Read the model definition and answer for the solid it produces. Units are mm, in the model's axes. Coordinates: 2 decimals unless noted, no trailing zeros. Write each loop counter-clockwise with the first axis right and the second up, starting at its lowest first coordinate (ties: lowest second). Pieces come first, ordered by that corner, then holes.
(1) Section D-D on z = 9 is taken. Write down the section's boundary in (x, y).
(2) Section C-C on y = -1.2 is taken. Write down the section's boundary in (x, z).
(3) Find the intervals of material crossed by probe 1 along X at (y, z) = (-0.7, 5); probe 2 along X at (y, z) = (1.25, 5.75); probe 3 along Z at (x, y) = (-10, -0.1), in increasing order.
(4) The mould has two halves that part along Z. Classify faces 1 (the cylindrical face through (8.753, -0.021, 3.373)), 2 (the flat face through (0, 0, 10)), 3 (the flat face through (0, 0, 0)), 4 (the cylindrical face through (0.09, -0.02, 2.95)): +Z half, -Z half, draft (parallel to the pull), parting line (faces both ways), or undercut.
(5) Given pin 1 (1.5 mm diameter, centred on y = 0, z = 6.5, fed in from -X); pin 2 (5.5 mm diameter, centred on x = 0, z = 5, fed in from +Y); pin 3 (3.5 mm diameter, centred on x = 10, z = 5, fed in from +Y), each flat-ended and moving along its own axis, determine where each tip first touches the part or whether it passes through.
(6) Section A-A on z = 5 is taken. Write down the section's boundary in (x, y).
(7) Section B-B on x = 0 is taken. Write down the section's boundary in (y, z).
from build123d import *

# Parameters (mm, degrees)
SKETCH1_R           = 2.05
BOSS_EXTRUDE1_DEPTH = 1.5


with BuildPart() as part:
    # Sketch1 → Boss-Extrude1 (new, symmetric)
    with BuildSketch(Plane(origin=(0, 0, 0), x_dir=(1, 0, 0), z_dir=(0, 1, 0))):
        with BuildLine():
            Line((-10, 0), (-5, 0))
            Line((-5, 0), (5, 0))
            Line((5, 0), (10, 0))
            ThreePointArc((10, 0), (15, -5), (10, -10))
            Line((10, -10), (5, -10))
            Line((5, -10), (-5, -10))
            Line((-5, -10), (-10, -10))
            ThreePointArc((-10, -10), (-15, -5), (-10, 0))
        make_face()
        with Locations(Location((10, -5, 0), (0, 0, 270))):
            Circle(SKETCH1_R, mode=Mode.SUBTRACT)
        with Locations(Location((-10, -5, 0), (0, 0, 90))):
            Circle(SKETCH1_R, mode=Mode.SUBTRACT)
        with Locations(Location((0, -5, 0), (0, 0, 270))):
            Circle(SKETCH1_R, mode=Mode.SUBTRACT)
    extrude(amount=BOSS_EXTRUDE1_DEPTH, both=True)


solid = part.part
Response:
1. outline: (-13, -1.5) - (13, -1.5) - (13, 1.5) - (-13, 1.5) - close
2. outline: (-10, 0) - (10, 0) arc R5 ccw to (10, 10) - (-10, 10) arc R5 ccw to start; hole circle Ø4.1 at (-10, 5); hole circle Ø4.1 at (0, 5); hole circle Ø4.1 at (10, 5)
3. probe 1: x = -15 to -12.05, -7.95 to -2.05, 2.05 to 7.95, 12.05 to 15
3. probe 2: x = -14.94 to -11.91, -8.09 to -1.91, 1.91 to 8.09, 11.91 to 14.94
3. probe 3: z = 0 to 2.95, 7.05 to 10
4. face 1: undercut
4. face 2: +Z half
4. face 3: -Z half
4. face 4: undercut
5. pin 1: stops at x = -14.94
5. pin 2: stops at y = 1.5
5. pin 3: passes through
6. outline: (-15, -1.5) - (-12.05, -1.5) - (-12.05, 1.5) - (-15, 1.5) - close; (-7.95, -1.5) - (-2.05, -1.5) - (-2.05, 1.5) - (-7.95, 1.5) - close; (2.05, -1.5) - (7.95, -1.5) - (7.95, 1.5) - (2.05, 1.5) - close; (12.05, -1.5) - (15, -1.5) - (15, 1.5) - (12.05, 1.5) - close
7. outline: (-1.5, 0) - (1.5, 0) - (1.5, 2.95) - (-1.5, 2.95) - close; (-1.5, 7.05) - (1.5, 7.05) - (1.5, 10) - (-1.5, 10) - close
